Part model, mm, in its own coordinate system. A direction names the side the tool comes from. Give positions to 0.01 mm unless a question says otherwise; leave off trailing zeros. Write each loop counter-clockwise with the first axis right and the second up, starting at its lowest first coordinate (ties: lowest second). Pieces come first, ordered by that corner, then holes. Notation, with made-up numbers: M 58,23.25 L 103,23.25 A17 ccw 103,35.25 Z; hole C 42,-21.75 d3. An arc over 180 degrees is marked long. Use CSV: the item, a comma, the result in double quotes. Start each with the question number.
1. Drop flat-ended pins along their axis: pin 1 Ø1 at (y, z) = (-69, 1.5) entering from -X; pin 2 Ø0.9 at (x, z) = (16.5, 1) entering from -Y; pin 3 Ø1.5 at (y, z) = (-44, 1) entering from +X. Give the stop position or say it passes through.
2. Band-saw the part on A-A, the plane x = 45.34. List the corners of the cut face in (y, z), then the cut area to 3 significant figures.
3. Band-saw the part on D-D, the plane z = 1.85. Count the separate pieces of the cut face and the enclosed holes in it, then the cut area to 3 significant figures.
4. Band-saw the part on B-B, the plane y = -10. List the corners of the cut face in (x, z).
5. Mould opens along X. For faces 4 (the face through (39, -59, 1)), 5 (the face through (56.54, -44.48, 1.52)), 6 (the face through (17, -18, 1)) say: pulls with the +X half, pulls with the -X half, needs draft (parallel to the pull), parting line crosses it, or undercut.
6. Band-saw the part on C-C, the plane x = 20. List the corners of the cut face in (y, z).
7. Drill centre lines: line 1 along Y through (x, z) = (69, 0.9); line 2 along Y through (x, z) = (60, 2.2); line 3 along Y through (x, z) = (78.5, 1.75). Where is each one in solid material? Low to high. Write a range as from..to.
8. 3-axis set-ups, long thin cutter, end or side, ignore diameter. For faces 1 (the face through (34, -22, 1)), 2 (the face through (75.034, -50.183, 1.521)), 3 (the face through (59, -35, 3)): which of +Z, -Z, +X, -X, +Y, -Y reach the whole face in a straight line?
from build123d import *

# Parameters (mm, degrees)
EXTRUDE_1_DEPTH     = 3
SKETCH_2_R          = 1.65
CUT_EXTRUDE_1_DEPTH = 148.059131493
CUT_EXTRUDE_2_DEPTH = 10


with BuildPart() as part:
    # 草图1 → 凸台-拉伸1 (new body)
    with BuildSketch(Plane.XY):
        Polygon((0, 0), (70, 0), (115.710678119, -45.710678119), (70.710678119, -90.710678119), (0, -20), align=None)
    extrude(amount=EXTRUDE_1_DEPTH)

    # 草图2 → 切除-拉伸1 (cut, through all)
    with BuildSketch(Plane.XY.offset(3)):
        with Locations((72.124891681, -75.154328933)):
            Circle(SKETCH_2_R)
        with Locations((97.580735804, -49.69848481)):
            Circle(SKETCH_2_R)
        with Locations((20, -10)):
            Circle(SKETCH_2_R)
        with Locations((45.34, -10)):
            Circle(SKETCH_2_R)
        with Locations((60, -10)):
            Circle(SKETCH_2_R)
        with Locations((73.729886297, -27.233840149)):
            Circle(SKETCH_2_R)
        with Locations((52.233840149, -48.729886297)):
            Circle(SKETCH_2_R)
        with Locations(Location((84.690041405, -38.193995257, 0), (0, 0, 180))):
            Circle(SKETCH_2_R)
        with Locations(Location((63.193995257, -59.690041405, 0), (0, 0, 180))):
            Circle(SKETCH_2_R)
        with Locations((84.852813742, -62.426406871)):
            Circle(SKETCH_2_R)
        with BuildLine():
            Line((56.511836175, -42.118437893), (67.118437893, -31.511836175))
            ThreePointArc((67.118437893, -31.511836175), (69.451890271, -31.511836175), (69.451890271, -33.845288553))
            Line((69.451890271, -33.845288553), (58.845288553, -44.451890271))
            ThreePointArc((58.845288553, -44.451890271), (56.511836175, -44.451890271), (56.511836175, -42.118437893))
        make_face()
        with BuildLine():
            Line((69.805443661, -55.412045379), (80.412045379, -44.805443661))
            ThreePointArc((80.412045379, -44.805443661), (80.412045379, -42.471991283), (78.078593001, -42.471991283))
            Line((78.078593001, -42.471991283), (67.471991283, -53.078593001))
            ThreePointArc((67.471991283, -53.078593001), (67.471991283, -55.412045379), (69.805443661, -55.412045379))
        make_face()
    extrude(amount=-CUT_EXTRUDE_1_DEPTH, mode=Mode.SUBTRACT)

    # 草图3 → 切除-拉伸2 (cut)
    with BuildSketch(Plane(origin=(0, 0, 0), x_dir=(-1, 0, 0), z_dir=(0, 0, -1))):
        Polygon((-34, -18), (2, -18), (-6, -26), (-34, -26), align=None)
    extrude(amount=-CUT_EXTRUDE_2_DEPTH, mode=Mode.SUBTRACT)


solid = part.part
Output:
1,pin 1,"stops at x = 48.5"
1,pin 2,"stops at y = -36.95"
1,pin 3,"stops at x = 114.75"
2,outline,"M -65.34,0 L -11.65,0 L -11.65,3 L -65.34,3 Z; M -8.35,0 L 0,0 L 0,3 L -8.35,3 Z"
2,area,"186 mm²"
3,separate pieces,"1"
3,enclosed holes,"12"
3,area,"5,480 mm²"
4,outline,"M 0,0 L 18.35,0 L 18.35,3 L 0,3 Z; M 21.65,0 L 43.69,0 L 43.69,3 L 21.65,3 Z; M 46.99,0 L 58.35,0 L 58.35,3 L 46.99,3 Z; M 61.65,0 L 80,0 L 80,3 L 61.65,3 Z"
5,face 4,"pulls with the -X half"
5,face 5,"undercut"
5,face 6,"needs draft"
6,outline,"M -40,0 L -26,0 L -26,3 L -40,3 Z; M -18,0 L -11.65,0 L -11.65,3 L -18,3 Z; M -8.35,0 L 0,0 L 0,3 L -8.35,3 Z"
7,line 1,"y = -89..-55.86, -51.55..-34.3, -31.19..0"
7,line 2,"y = -80..-43.3, -38.63..-11.65, -8.35..0"
7,line 3,"y = -82.92..-46.72, -42.17..-8.5"
8,face 1,"+Z, -Z, -X"
8,face 2,"+Z, -Z"
8,face 3,"+Z, +X, -X, +Y, -Y"
